Can you work these out from the model? Positions are in its coordinate system, mm. Face numbers are marked on the shaded views. Round coordinates to 2 decimals unless told otherwise and drop trailing zeros. Order: outer loops, then holes, each group sorted by start corner. A loop starts at its lowest first (then second) coordinate and runs counter-clockwise, first axis right, second up. Notation, with made-up numbers: M -3.5,-32.75 L 14.5,-32.75 A12 cw 14.5,-20.75 Z; hole C 18.5,-36.75 d7. An arc over 180 degrees is marked long. One line per question, with ' | ' between items.
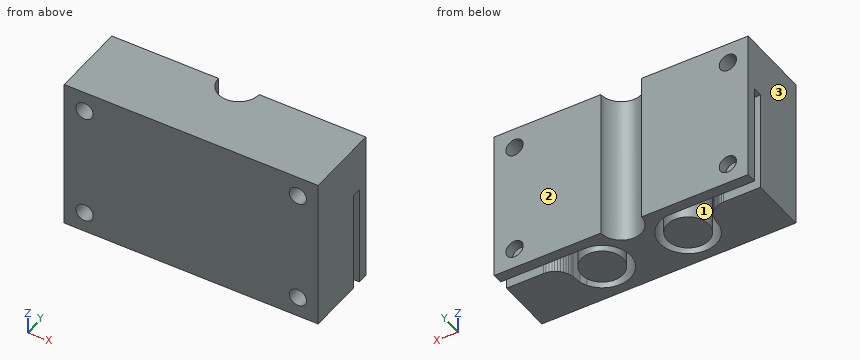
```python
from build123d import *

# Parameters (mm, degrees)
SCHIZZO1_W                   = 50
SCHIZZO1_H                   = 15
ESTRUSIONE_ESTRUSIONE1_DEPTH = 30
SCHIZZO2_R                   = 4.08343654
TAGLIO_ESTRUSIONE1_DEPTH     = 20
SCHIZZO6_R                   = 1.7
TAGLIO_ESTRUSIONE3_DEPTH     = 30
SCHIZZO9_R                   = 4
TAGLIO_ESTRUSIONE5_DEPTH     = 64.492497112


with BuildPart() as part:
    # Schizzo1 → Estrusione-Estrusione1 (new body)
    with BuildSketch(Plane.XY):
        with Locations((25, 17.625628141)):
            Rectangle(SCHIZZO1_W, SCHIZZO1_H)
    extrude(amount=ESTRUSIONE_ESTRUSIONE1_DEPTH)

    # Schizzo2 → Taglio-Estrusione1 (cut)
    # profile 1 of 2: a face of its own
    with BuildSketch(Plane.XY):
        with BuildLine():
            ThreePointArc((16.544218644, 23.125628141), (21.393626777, 14.807370827), (11.765784724, 14.685627772))
            Line((11.765784724, 14.685627772), (11.214334392, 16.016946643))
            Line((11.214334392, 16.016946643), (10.994077631, 17.936406255))
            Line((10.994077631, 17.936406255), (10.89812606, 18.418787382))
            Line((10.89812606, 18.418787382), (10.740031995, 18.884517478))
            Line((10.740031995, 18.884517478), (10.522500471, 19.325627772))
            Line((10.522500471, 19.325627772), (10.249253512, 19.734570745))
            Line((10.249253512, 19.734570745), (9.92496645, 20.10434927))
            Line((9.92496645, 20.10434927), (9.555187926, 20.428636332))
            Line((9.555187926, 20.428636332), (9.146244953, 20.701883291))
            Line((9.146244953, 20.701883291), (8.705134658, 20.919414815))
            Line((8.705134658, 20.919414815), (8.239404562, 21.077508879))
            Line((8.239404562, 21.077508879), (7.757023435, 21.173460451))
            Line((7.757023435, 21.173460451), (7.266244953, 21.205627772))
            Line((7.266244953, 21.205627772), (-0.789507737, 21.205627772))
            Line((-0.789507737, 21.205627772), (-0.789507737, 23.125628141))
            Line((-0.789507737, 23.125628141), (16.544218644, 23.125628141))
        make_face()
        with Locations((16.544218644, 17.552936622)):
            Circle(SCHIZZO2_R, mode=Mode.SUBTRACT)
    # profile 2 of 2: a face of its own
    with BuildSketch(Plane.XY):
        with BuildLine():
            Line((33.455781356, 23.125628141), (50.789507737, 23.125628141))
            Line((50.789507737, 23.125628141), (50.789507737, 21.205627772))
            Line((50.789507737, 21.205627772), (42.733755047, 21.205627772))
            Line((42.733755047, 21.205627772), (42.242976565, 21.173460451))
            Line((42.242976565, 21.173460451), (41.760595438, 21.077508879))
            Line((41.760595438, 21.077508879), (41.294865342, 20.919414815))
            Line((41.294865342, 20.919414815), (40.853755047, 20.701883291))
            Line((40.853755047, 20.701883291), (40.444812074, 20.428636332))
            Line((40.444812074, 20.428636332), (40.07503355, 20.10434927))
            Line((40.07503355, 20.10434927), (39.750746488, 19.734570745))
            Line((39.750746488, 19.734570745), (39.477499529, 19.325627772))
            Line((39.477499529, 19.325627772), (39.259968005, 18.884517478))
            Line((39.259968005, 18.884517478), (39.10187394, 18.418787382))
            Line((39.10187394, 18.418787382), (39.005922369, 17.936406255))
            Line((39.005922369, 17.936406255), (38.785665608, 16.016946643))
            Line((38.785665608, 16.016946643), (38.234215276, 14.685627772))
            ThreePointArc((38.234215276, 14.685627772), (28.606373223, 14.807370827), (33.455781356, 23.125628141))
        make_face()
        with Locations((33.455781356, 17.552936622)):
            Circle(SCHIZZO2_R, mode=Mode.SUBTRACT)
    extrude(amount=TAGLIO_ESTRUSIONE1_DEPTH, mode=Mode.SUBTRACT)

    # Schizzo6 → Taglio-Estrusione3 (cut)
    with BuildSketch(Plane(origin=(0, 25.125628141, 0), x_dir=(1, 0, 0), z_dir=(0, 1, 0))):
        with Locations(Location((4, -4, 0), (0, 0, 270))):
            Circle(SCHIZZO6_R)
        with Locations(Location((46, -4, 0), (0, 0, 270))):
            Circle(SCHIZZO6_R)
        with Locations(Location((46, -26, 0), (0, 0, 270))):
            Circle(SCHIZZO6_R)
        with Locations(Location((4, -26, 0), (0, 0, 270))):
            Circle(SCHIZZO6_R)
    extrude(amount=-TAGLIO_ESTRUSIONE3_DEPTH, mode=Mode.SUBTRACT)

    # Schizzo9 → Taglio-Estrusione5 (cut, through all)
    with BuildSketch(Plane(origin=(0, 0, 0), x_dir=(-1, 0, 0), z_dir=(0, 0, -1))):
        with Locations((-25, 25.125628141)):
            Circle(SCHIZZO9_R)
    extrude(amount=-TAGLIO_ESTRUSIONE5_DEPTH, mode=Mode.SUBTRACT)


solid = part.part
```
(1) If we section it at B-B on x = 46: Please give me the cut outline in (y, z).
Final values:
outline: M 10.13,0 L 21.21,0 L 21.21,2.3 L 10.13,2.3 Z; M 10.13,5.7 L 21.21,5.7 L 21.21,20 L 23.13,20 L 23.13,5.7 L 25.13,5.7 L 25.13,24.3 L 10.13,24.3 Z; M 10.13,27.7 L 25.13,27.7 L 25.13,30 L 10.13,30 Z; M 23.13,0 L 25.13,0 L 25.13,2.3 L 23.13,2.3 Z
(2) Thinking about a two-plate mould opening in Y: for the marked faces 1, 2 and 3, which applies, released by +Y, released by -Y, zero draft, split by the parting line, or undercut?
Final values:
face 1: undercut | face 2: released by +Y | face 3: zero draft
(3) If we section it at D-D on x = 14: Please give me the cut outline in (y, z).
Final values:
outline: M 10.13,0 L 12.59,0 L 12.59,20 L 14.36,20 L 14.36,0 L 20.75,0 L 20.75,20 L 23.13,20 L 23.13,0 L 25.13,0 L 25.13,30 L 10.13,30 Z
(4) If we section it at C-C on y = 23.75: Please give me the cut outline in (x, z), plus the area to 3 significant figures.
Final values:
outline: M 0,0 L 21.24,0 L 21.24,30 L 0,30 Z; M 28.76,0 L 50,0 L 50,30 L 28.76,30 Z; hole C 4,4 d3.4; hole C 4,26 d3.4; hole C 46,4 d3.4; hole C 46,26 d3.4 | area: 1,240 mm^2
(5) Please list where these lines run through material, in increasing order: probe 1 along Y at (x, z) = (2, 13); probe 2 along X at (y, z) = (17.25, 9.25); probe 3 along X at (y, z) = (18.75, 6.5). Write a range as [from, to].
Final values:
probe 1: [10.13, 21.21], [23.13, 25.13] | probe 2: [0, 11.07], [12.47, 20.62], [22.11, 27.89], [29.38, 37.53], [38.93, 50] | probe 3: [0, 10.79], [12.64, 20.45], [21.99, 28.01], [29.55, 37.36], [39.21, 50]
(6) If we section it at A-A on z = 26: Please give me the cut outline in (x, y).
Final values:
outline: M 0,10.13 L 2.3,10.13 L 2.3,25.13 L 0,25.13 Z; M 5.7,10.13 L 44.3,10.13 L 44.3,25.13 L 29,25.13 A4 cw 21,25.13 L 5.7,25.13 Z; M 47.7,10.13 L 50,10.13 L 50,25.13 L 47.7,25.13 Z
